Work out the finished part from the listing and answer in its coordinate system (mm). A direction names the side the tool comes from. Round coordinates to 2 decimals unless told otherwise and drop trailing zeros. Order: outer loops, then holes, each group sorted by start corner. A loop starts at its lowest first (then second) coordinate and runs counter-clockwise, first axis right, second up. Notation, with made-up numbers: M 61.25,0 L 104.25,0 A19 ccw 104.25,26 Z; hole C -39,-20 d2. An arc over 180 degrees is marked long. Answer as a JSON object with one key per item and string values. Group by question number.
from build123d import *

# Parameters (mm, degrees)
SKETCH1_R                = 13.75
BOSS_EXTRUDE1_DEPTH      = 9.5
SKETCH2_W                = 44.25
SKETCH2_H                = 20
BOSS_EXTRUDE2_DEPTH      = 9.5
BOSS_EXTRUDE3_REACH      = 49.301
BOSS_EXTRUDE3_END_RADIUS = 16.25
SKETCH3_R                = 2
SKETCH4_W                = 25
SKETCH4_H                = 7
CUT_EXTRUDE1_DEPTH       = 1
CUT_EXTRUDE2_DEPTH       = 48.300898561
FILLET1_R                = 1


with BuildPart() as part:
    # Sketch1 → Boss-Extrude1 (new body)
    with BuildSketch(Plane(origin=(0, 0, 0), x_dir=(1, 0, 0), z_dir=(0, 1, 0))):
        with Locations(Location((0, 0, 0), (0, 0, 270))):
            Circle(SKETCH1_R)
    extrude(amount=BOSS_EXTRUDE1_DEPTH)

    # Sketch2 → Boss-Extrude2 (add)
    with BuildSketch(Plane(origin=(0, 0, 0), x_dir=(1, 0, 0), z_dir=(0, 1, 0))):
        with Locations((22.125, 0)):
            Rectangle(SKETCH2_W, SKETCH2_H)
    extrude(amount=BOSS_EXTRUDE2_DEPTH)

    # Boss-Extrude3: up to this cylinder (the profile starts inside it)
    boss_extrude3_end = Plane(origin=(0, 4.5, 0), z_dir=(0, -1, 0)) * Cylinder(BOSS_EXTRUDE3_END_RADIUS, 132.102, mode=Mode.PRIVATE)
    # Sketch3 → Boss-Extrude3 (add, up to the surface)
    with BuildSketch(Plane(origin=(0, 0, 0), x_dir=(0, 0, -1), z_dir=(1, 0, 0)), mode=Mode.PRIVATE) as boss_extrude3_sk1:
        with Locations((0, 4.5)):
            Circle(SKETCH3_R)
    boss_extrude3_tool1 = extrude(boss_extrude3_sk1.sketch, amount=-BOSS_EXTRUDE3_REACH, mode=Mode.PRIVATE) & boss_extrude3_end
    add(boss_extrude3_tool1.solids().sort_by_distance((0, 4.5, 0))[0])

    # Sketch4 → Cut-Extrude1 (cut)
    with BuildSketch(Plane(origin=(0, 9.5, 0), x_dir=(1, 0, 0), z_dir=(0, 1, 0))):
        with Locations((26.75, 0)):
            Rectangle(SKETCH4_W, SKETCH4_H)
    extrude(amount=-CUT_EXTRUDE1_DEPTH, mode=Mode.SUBTRACT)

    # Sketch5 → Cut-Extrude2 (cut, through all)
    with BuildSketch(Plane(origin=(0, 9.5, 0), x_dir=(1, 0, 0), z_dir=(0, 1, 0))):
        with BuildLine():
            Line((42.75, 10), (47.75, 10))
            Line((47.75, 10), (47.75, -10))
            Line((47.75, -10), (42.75, -10))
            ThreePointArc((42.75, -10), (44.25, 0), (42.75, 10))
        make_face()
    extrude(amount=-CUT_EXTRUDE2_DEPTH, mode=Mode.SUBTRACT)

    # Fillet1
    fillet1_edges = [part.edges().sort_by_distance(p)[0] for p in [
        (42.75, 4.75, 10),
        (42.75, 4.75, -10),
    ]]
    fillet(fillet1_edges, radius=FILLET1_R)


solid = part.part
Item 1: Consider L1, parallel to Z at x = 36, y = 8.75; L2, parallel to Z at x = 30, y = 0.75; L3, parallel to X at y = 2, z = -12.25 (3 decimals). Determine where each line is inside the solid, lowest interval first.
Item 2: Each of these flat-tipped pins is pushed along its axis until it touches: pin 1 (3 mm diameter, centred on x = 23.5, y = 4, fed in from -Z); pin 2 (8 mm diameter, centred on x = 36.5, z = -2, fed in from +Y); pin 3 (4 mm diameter, centred on y = 4, z = 7, fed in from -X); pin 4 (0.5 mm diameter, centred on x = 31, y = 9, fed in from +Z). Where does it stop, or does it pass through?
Item 3: Find section A-A (y = 4.5). Give the vertices of the cut face in (x, z), and give its area (3 significant figures).
Item 4: The mould has two halves that part along X. Classify faces 1 (the flat face through (27, 8.5, 0)), 2 (the cylindrical face through (-13.743, 6.795, -0.448)), 3 (the flat face through (16, 0, 0)), 4 (the cylindrical face through (44.25, 4.82, 0.13)): +X half, -X half, draft (parallel to the pull), parting line (faces both ways), or undercut.
Item 5: Find section D-D (y = 1). Give the vertices of the cut face in (x, z).
Item 6: A tool of negligible diameter and unlimited length cuts with its end or side. For faces 5 (the flat face through (9, 9.5, 0)), 6 (the cylindrical face through (-14.908, 3.734, -1.847)), 7 (the flat face through (25, 5, -10)), 8 (the flat face through (25, 5, 10)), 9 (the cylindrical face through (-16.25, 4.47, 0.04)), from which of +Z, -Z, +X, -X, +Y, -Y can it reach the whole face along a straight path? Write none if from no direction.
Item 7: Find section B-B (z = 0). Give the vertices of the cut face in (x, y), and give its area (3 significant figures).
Item 8: Find section C-C (x = -5). Give the vertices of the cut face in (y, z), and give its area (3 significant figures).
Responses:
{
 "1": {"L1": "z = -10 to -3.5, 3.5 to 10", "L2": "z = -10 to 10", "L3": "x = -6.245 to 6.245"},
 "2": {"pin 1": "stops at z = -10", "pin 2": "stops at y = 9.5", "pin 3": "stops at x = -12.81", "pin 4": "stops at z = 10"},
 "3": {"outline": "M -16.13,-2 L -13.6,-2 A13.75 ccw 9.44,-10 L 42,-10 A1 ccw 42.96,-9.27 A34.08 ccw 42.96,9.27 A1 ccw 42,10 L 9.44,10 A13.75 ccw -13.6,2 L -16.13,2 A16.25 ccw Z", "area": "1,230 mm^2"},
 "4": {"face 1": "undercut", "face 2": "parting line", "face 3": "draft", "face 4": "+X half"},
 "5": {"outline": "M 9.44,-10 L 42,-10 A1 ccw 42.96,-9.27 A34.08 ccw 42.96,9.27 A1 ccw 42,10 L 9.44,10 A13.75 ccw long Z"},
 "6": {"face 5": "+Z, -Z, +X, -X, +Y", "face 6": "-X", "face 7": "-Z, +X, +Y, -Y", "face 8": "+Z, +X, +Y, -Y", "face 9": "-X, +Y, -Y"},
 "7": {"outline": "M -16.25,2.5 L -13.75,2.5 L -13.75,0 L 44.25,0 L 44.25,9.5 L 39.25,9.5 L 39.25,8.5 L 14.25,8.5 L 14.25,9.5 L -13.75,9.5 L -13.75,6.5 L -16.25,6.5 Z", "area": "536 mm^2"},
 "8": {"outline": "M 0,-12.81 L 9.5,-12.81 L 9.5,12.81 L 0,12.81 Z", "area": "243 mm^2"}
}
